Check sheet for the drawn part. Datum: minimum x, y, z corner. Units: mm. Coordinates: 2 decimals unless noted, no trailing zeros. Write each loop counter-clockwise with the first axis right and the second up, starting at its lowest first coordinate (ties: lowest second). Pieces come first, ordered by that corner, then holes. Notation, with made-up numbers: (51, -18) -> (77, -18) arc R29 cw to (77, 8) -> close; hole circle Ø6 at (-6, 42). An arc over 180 degrees is marked (long way). Answer in a Markdown table with one row per item. Add a question column.
1. Cross-section at A-A on x = 100. Record the cut outline in (y, z), and give its area (3 significant figures).
2. Cross-section at C-C on y = 4.9. Give the number of separate pieces and of enclosed holes in the cut face, and give its area (3 significant figures).
3. Cross-section at B-B on z = 35. Record the cut outline in (x, y).
4. Cross-section at D-D on x = 31. Record the cut outline in (y, z).
5. Scan lines: L1, parallel to X at y = 4.5, z = 180; L2, parallel to Z at x = 100, y = 1.25; L3, parallel to Z at x = 47.5, y = 2.2. Record each from-to range of solid material in increasing order. Write a range as from..to.
6. Depth check by flat-ended pin: P1, Ø6, axis at x = 100, z = 35, coming from the -Y side; P2, Ø1.8, axis at y = 4.5, z = 61, coming from the -X side; P3, Ø1, axis at y = 5, z = 78, coming from the +X side; P4, Ø3, axis at y = 3.5, z = 4, coming from the +X side. Enter the tip coordinate at first touch or a pass-through.
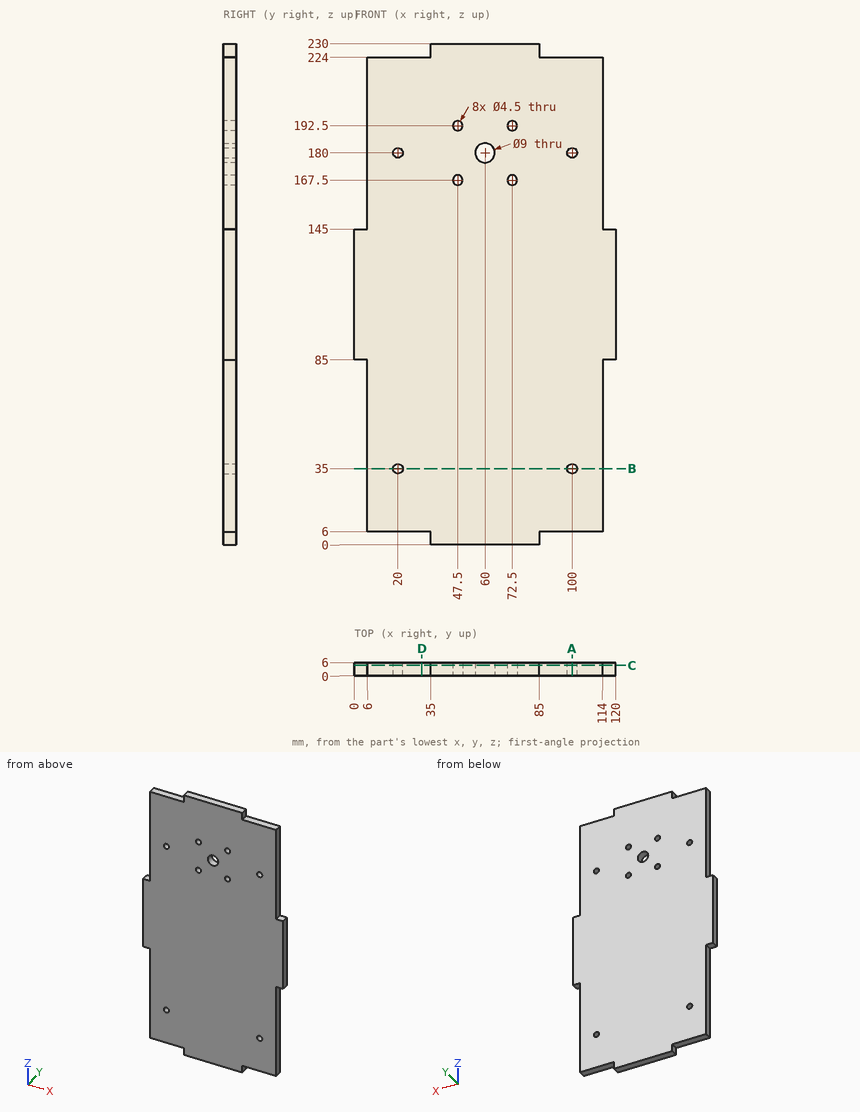
Results found:
| question | item | result |
|---|---|---|
| 1 | outline | (0, 6) -> (6, 6) -> (6, 32.75) -> (0, 32.75) -> close; (0, 37.25) -> (6, 37.25) -> (6, 177.75) -> (0, 177.75) -> close; (0, 182.25) -> (6, 182.25) -> (6, 224) -> (0, 224) -> close |
| 1 | area | 1,250 mm^2 |
| 2 | separate pieces | 1 |
| 2 | enclosed holes | 9 |
| 2 | area | 24,700 mm^2 |
| 3 | outline | (6, 0) -> (17.75, 0) -> (17.75, 6) -> (6, 6) -> close; (22.25, 0) -> (97.75, 0) -> (97.75, 6) -> (22.25, 6) -> close; (102.25, 0) -> (114, 0) -> (114, 6) -> (102.25, 6) -> close |
| 4 | outline | (0, 6) -> (6, 6) -> (6, 224) -> (0, 224) -> close |
| 5 | L1 | x = 6..17.75, 22.25..55.5, 64.5..97.75, 102.25..114 |
| 5 | L2 | z = 6..32.75, 37.25..177.75, 182.25..224 |
| 5 | L3 | z = 0..165.25, 169.75..190.25, 194.75..230 |
| 6 | P1 | stops at y = 0 |
| 6 | P2 | stops at x = 6 |
| 6 | P3 | stops at x = 114 |
| 6 | P4 | stops at x = 85 |
